The figure shows three views and two pictorial views of one solid part (mm, origin at its lowest corner). Answer the questions. A direction names the side the tool comes from. Give positions to 0.01 mm unless a question says otherwise; leave off trailing zeros. Order: outer loops, then holes, each group sorted by start corner. A loop starts at its lowest first (then second) coordinate and runs counter-clockwise, first axis right, second up. Notation, with made-up numbers: (-29.5, 74) - (-24.5, 74) arc R23 cw to (-24.5, 108) - close; hole circle Ø1 at (39.25, 37). An arc over 180 degrees is marked (long way). Use a Markdown table: item, result. Add a question column.
1. A cutting plane is placed at A-A on z = 73. Determine the outline of the cut face in (x, y).
2. A cutting plane is placed at C-C on y = 35.25. State how many separate pieces and enclosed holes the cut face has, and give its area (3 significant figures).
3. Flat-ended cylindrical pins translate along their axes: P1, Ø3, axis at x = 25, y = 10, coming from the -Z side; P2, Ø1.7, axis at y = 11, z = 29, coming from the +X side; P3, Ø6.5, axis at y = 35.5, z = 29.5, coming from the +X side; P4, Ø1, axis at x = 13, y = 27, coming from the +Z side. Find the tip coordinate at first contact, or state that the pin passes through.
4. A cutting plane is placed at B-B on x = 15. Determine the outline of the cut face in (y, z).
5. Which of the six approach directions +Z, -Z, +X, -X, +Y, -Y give full straight-line access (tool end or side, diameter ignored) to the marked faces 1 and 2?
6. Consider L1, parallel to Z at x = 4.5, y = 9.75; L2, parallel to Z at x = 7.8, y = 35.25; L3, parallel to Y at x = 2.25, z = 73. Determine where each line is inside the solid, lowest interval first.
7. A cutting plane is placed at D-D on y = 29.5. Determine the outline of the cut face in (x, z).
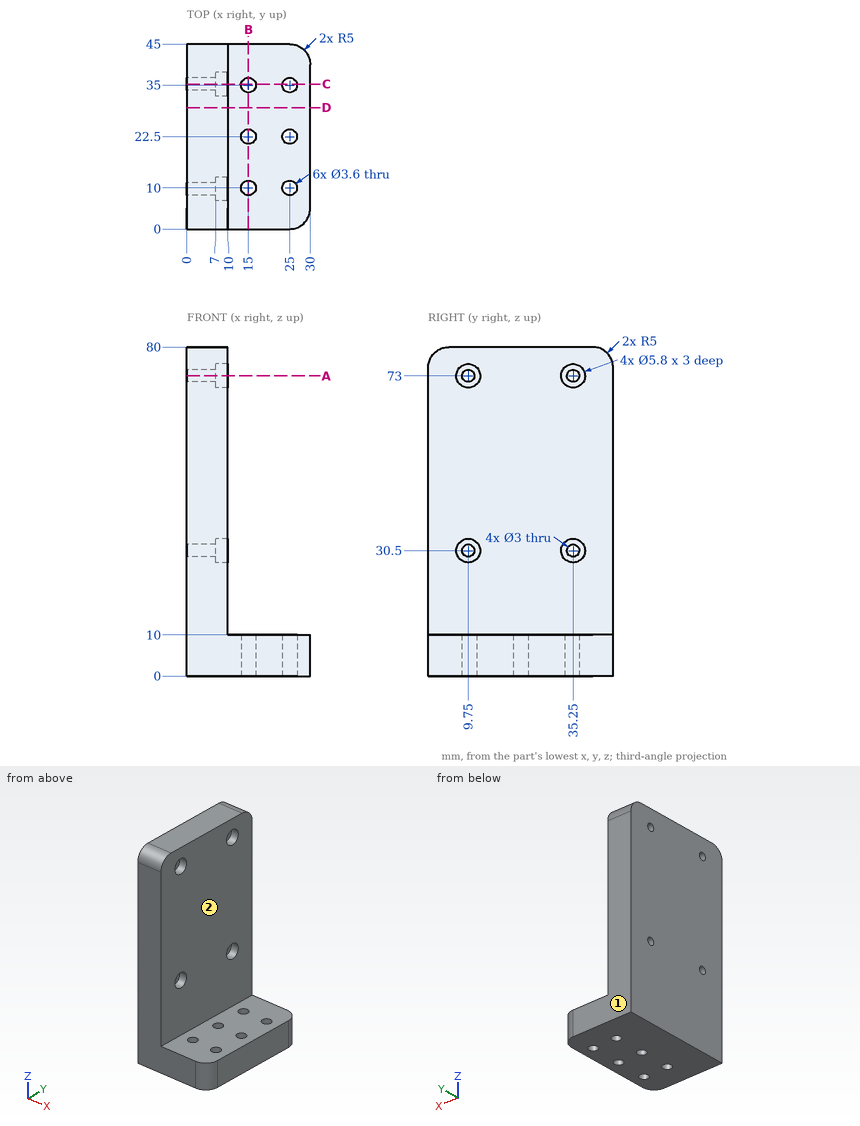
Output values:
| question | item | result |
|---|---|---|
| 1 | outline | (0, 0) - (10, 0) - (10, 6.85) - (7, 6.85) - (7, 8.25) - (0, 8.25) - close; (0, 11.25) - (7, 11.25) - (7, 12.65) - (10, 12.65) - (10, 32.35) - (7, 32.35) - (7, 33.75) - (0, 33.75) - close; (0, 36.75) - (7, 36.75) - (7, 38.15) - (10, 38.15) - (10, 45) - (0, 45) - close |
| 2 | separate pieces | 5 |
| 2 | enclosed holes | 0 |
| 2 | area | 852 mm² |
| 3 | P1 | through |
| 3 | P2 | x = 7 |
| 3 | P3 | x = 10 |
| 3 | P4 | z = 10 |
| 4 | outline | (0, 0) - (8.2, 0) - (8.2, 10) - (0, 10) - close; (11.8, 0) - (20.7, 0) - (20.7, 10) - (11.8, 10) - close; (24.3, 0) - (33.2, 0) - (33.2, 10) - (24.3, 10) - close; (36.8, 0) - (45, 0) - (45, 10) - (36.8, 10) - close |
| 5 | face 1 | +Z, -Z, +X, -X, +Y |
| 5 | face 2 | +Z, +X, +Y, -Y |
| 6 | L1 | 0 to 29, 32 to 71.5, 74.5 to 80 |
| 6 | L2 | 0 to 27.6, 33.4 to 70.1, 75.9 to 80 |
| 6 | L3 | 0 to 8.25, 11.25 to 33.75, 36.75 to 45 |
| 7 | outline | (0, 0) - (30, 0) - (30, 10) - (10, 10) - (10, 80) - (0, 80) - close |
